from build123d import *

# Parameters (mm, degrees)
SKETCH1_W           = 80
SKETCH1_H           = 50
BOSS_EXTRUDE1_DEPTH = 6
SKETCH4_W           = 52.5
SKETCH4_H           = 30.8
SKETCH4_W_2         = 42.5
SKETCH4_H_2         = 20.8
BOSS_EXTRUDE2_DEPTH = 10
SKETCH5_W           = 5
SKETCH5_H           = 8
CUT_EXTRUDE1_DEPTH  = 7.6
SKETCH6_R           = 1.15
CUT_EXTRUDE2_DEPTH  = 49.218253805
SKETCH7_R           = 2.1
CUT_EXTRUDE3_DEPTH  = 4.41
CHAMFER3_SIZE       = 1
CHAMFER4_SIZE       = 0.5
SKETCH8_R           = 2.25
CUT_EXTRUDE4_DEPTH  = 49.218253805
FILLET1_R           = 2
CHAMFER5_SIZE       = 1


with BuildPart() as part:
    # Sketch1 → Boss-Extrude1 (new body)
    with BuildSketch(Plane(origin=(0, 0, 0), x_dir=(1, 0, 0), z_dir=(0, 1, 0))):
        Rectangle(SKETCH1_W, SKETCH1_H)
    extrude(amount=BOSS_EXTRUDE1_DEPTH)

    # Sketch4 → Boss-Extrude2 (add)
    with BuildSketch(Plane(origin=(0, 6, 0), x_dir=(1, 0, 0), z_dir=(0, 1, 0))):
        with Locations((-10.25, 0)):
            Rectangle(SKETCH4_W, SKETCH4_H)
        with Locations((-10.25, 0)):
            Rectangle(SKETCH4_W_2, SKETCH4_H_2, mode=Mode.SUBTRACT)
    extrude(amount=BOSS_EXTRUDE2_DEPTH)

    # Sketch5 → Cut-Extrude1 (cut)
    with BuildSketch(Plane(origin=(0, 16, 0), x_dir=(1, 0, 0), z_dir=(0, 1, 0))):
        with Locations((13.5, 0)):
            Rectangle(SKETCH5_W, SKETCH5_H)
    extrude(amount=-CUT_EXTRUDE1_DEPTH, mode=Mode.SUBTRACT)

    # Sketch6 → Cut-Extrude2 (cut, through all)
    with BuildSketch(Plane(origin=(0, 6, 0), x_dir=(1, 0, 0), z_dir=(0, 1, 0))):
        with Locations(Location((-28.35, 7.7, 0), (0, 0, 270))):
            Circle(SKETCH6_R)
        with Locations(Location((7.85, 7.7, 0), (0, 0, 90))):
            Circle(SKETCH6_R)
        with Locations(Location((7.85, -7.7, 0), (0, 0, 270))):
            Circle(SKETCH6_R)
        with Locations(Location((-28.35, -7.7, 0), (0, 0, 90))):
            Circle(SKETCH6_R)
    extrude(amount=-CUT_EXTRUDE2_DEPTH, mode=Mode.SUBTRACT)

    # Sketch7 → Cut-Extrude3 (cut)
    with BuildSketch(Plane.XZ):
        with Locations(Location((-28.35, 7.7, 0), (0, 0, 270))):
            Circle(SKETCH7_R)
        with Locations(Location((7.85, 7.7, 0), (0, 0, 270))):
            Circle(SKETCH7_R)
        with Locations(Location((-28.35, -7.7, 0), (0, 0, 270))):
            Circle(SKETCH7_R)
        with Locations(Location((7.85, -7.7, 0), (0, 0, 270))):
            Circle(SKETCH7_R)
    extrude(amount=-CUT_EXTRUDE3_DEPTH, mode=Mode.SUBTRACT)

    # Chamfer3
    chamfer3_edges = [part.edges().sort_by_distance(p)[0] for p in [
        (16, 16, 9.7),
        (-10.25, 16, -15.4),
        (-36.5, 16, 0),
        (-10.25, 16, 15.4),
        (16, 11, 15.4),
        (16, 11, -15.4),
        (-36.5, 11, -15.4),
        (-36.5, 11, 15.4),
        (11, 16, 7.2),
        (-10.25, 16, -10.4),
        (-31.5, 16, 0),
        (-10.25, 16, 10.4),
        (11, 16, -7.2),
        (16, 16, -9.7),
        (16, 8.4, 0),
        (16, 12.2, -4),
        (16, 12.2, 4),
        (11, 8.4, 0),
        (11, 12.2, 4),
        (11, 12.2, -4),
        (13.5, 16, -4),
        (13.5, 16, 4),
    ]]
    chamfer(chamfer3_edges, length=CHAMFER3_SIZE)

    # Chamfer4
    chamfer4_edges = [part.edges().sort_by_distance(p)[0] for p in [
        (7.85, 0, 9.8),
        (-28.35, 0, -5.6),
        (7.85, 0, -5.6),
        (-28.35, 0, 9.8),
    ]]
    chamfer(chamfer4_edges, length=CHAMFER4_SIZE)

    # Sketch8 → Cut-Extrude4 (cut, through all)
    with BuildSketch(Plane(origin=(0, 6, 0), x_dir=(1, 0, 0), z_dir=(0, 1, 0))):
        with Locations(Location((-35.5, 20.5, 0), (0, 0, 270))):
            Circle(SKETCH8_R)
        with Locations(Location((35.5, 20.5, 0), (0, 0, 270))):
            Circle(SKETCH8_R)
        with Locations(Location((35.5, -20.5, 0), (0, 0, 270))):
            Circle(SKETCH8_R)
        with Locations(Location((-35.5, -20.5, 0), (0, 0, 270))):
            Circle(SKETCH8_R)
    extrude(amount=-CUT_EXTRUDE4_DEPTH, mode=Mode.SUBTRACT)

    # Fillet1
    fillet1_edges = [part.edges().sort_by_distance(p)[0] for p in [
        (40, 3, 25),
        (-40, 3, 25),
        (-40, 3, -25),
        (40, 3, -25),
    ]]
    fillet(fillet1_edges, radius=FILLET1_R)

    # Chamfer5
    chamfer5_edges = [part.edges().sort_by_distance(p)[0] for p in [
        (-40, 0, 0),
        (-40, 6, 0),
        (40, 0, 0),
        (0, 0, 25),
        (0, 0, -25),
        (-39.414213562, 0, 24.414213562),
        (39.414213562, 0, 24.414213562),
        (39.414213562, 0, -24.414213562),
        (-39.414213562, 0, -24.414213562),
        (0, 6, -25),
        (40, 6, 0),
        (0, 6, 25),
        (-39.414213562, 6, 24.414213562),
        (39.414213562, 6, 24.414213562),
        (39.414213562, 6, -24.414213562),
        (-39.414213562, 6, -24.414213562),
    ]]
    chamfer(chamfer5_edges, length=CHAMFER5_SIZE)


solid = part.part
CAD build for the part. Positions are in the model's coordinates, mm. A direction names the side the tool comes from. Round coordinates to 2 decimals unless told otherwise and drop trailing zeros. Write each loop counter-clockwise with the first axis right and the second up, starting at its lowest first coordinate (ties: lowest second). Pieces come first, ordered by that corner, then holes.
(1) Drop flat-ended pins along their axis: P1, Ø2.5, axis at x = -28.35, z = -7.7, coming from the +Y side; P2, Ø2.5, axis at x = -8, y = 12.5, coming from the -Z side; P3, Ø4.5, axis at x = 7, z = 8.5, coming from the -Y side; P4, Ø0.9, axis at x = 13.5, z = 0.5, coming from the +Y side. Give the stop position or say it passes through.
(2) 3-axis set-ups, long thin cutter, end or side, ignore diameter. For faces 4 (the face through (-11, 10, -15.4)), 5 (the face through (-11, 10, 10.4)), 6 (the face through (-29.3, 4.41, 6.8)): which of +Z, -Z, +X, -X, +Y, -Y reach the whole face in a straight line?
(3) Slice it at B-B, the plane z = 20.5. Write the cut outline in (x, y).
(4) Slice it at A-A, the plane x = 35.5. Write the cut outline in (y, z), and give its area (3 significant figures).
(5) Mould opens along Z. For faces 1 (the face through (-39.43, 3.03, 24.4)), 2 (the face through (6.9, 4.41, 6.8)), 3 (the face through (-36.5, 10, 0)) say: pulls with the +Z half, pulls with the -Z half, needs draft (parallel to the pull), parting line crosses it, or undercut.
(6) Probe line 1 along X through (y, z) = (2, -20.5); line 2 along X through (y, z) = (3.3, -7.7); line 3 along Z through (x, y) = (15, 15). List the from-to ranges inside material, lowest first.
(7) Slice it at D-D, the plane z = 0. Write the cut outline in (x, y).
(8) Slice it at C-C, the plane y = 2.25. Count the separate pieces of the cut face and the enclosed holes in it, and give its area (3 significant figures).
From the geometry:
1. P1: stops at y = 6
1. P2: stops at z = -15.4
1. P3: stops at y = 0
1. P4: stops at y = 8.4
2. face 4: -Z, +X, -X, +Y
2. face 5: +Y
2. face 6: -Y
3. outline: (-40, 1) - (-39, 0) - (-37.75, 0) - (-37.75, 6) - (-39, 6) - (-40, 5) - close; (-33.25, 0) - (33.25, 0) - (33.25, 6) - (-33.25, 6) - close; (37.75, 0) - (39, 0) - (40, 1) - (40, 5) - (39, 6) - (37.75, 6) - close
4. outline: (0, -24) - (1, -25) - (5, -25) - (6, -24) - (6, -22.75) - (0, -22.75) - close; (0, -18.25) - (6, -18.25) - (6, 18.25) - (0, 18.25) - close; (0, 22.75) - (6, 22.75) - (6, 24) - (5, 25) - (1, 25) - (0, 24) - close
4. area: 244 mm2
5. face 1: pulls with the +Z half
5. face 2: undercut
5. face 3: needs draft
6. line 1: x = -40 to -37.75, -33.25 to 33.25, 37.75 to 40
6. line 2: x = -40 to -30.45, -26.25 to 5.75, 9.95 to 40
6. line 3: z = -15.4 to -4, 4 to 15.4
7. outline: (-40, 1) - (-39, 0) - (39, 0) - (40, 1) - (40, 5) - (39, 6) - (16, 6) - (16, 7.4) - (15, 8.4) - (12, 8.4) - (11, 7.4) - (11, 6) - (-31.5, 6) - (-31.5, 15) - (-32.5, 16) - (-35.5, 16) - (-36.5, 15) - (-36.5, 6) - (-39, 6) - (-40, 5) - close
8. separate pieces: 1
8. enclosed holes: 8
8. area: 3,880 mm2
